Work out the finished part from the listing and answer in its coordinate system (mm). A direction names the side the tool comes from. Coordinates: 2 decimals unless noted, no trailing zeros. Order: outer loops, then holes, each group sorted by start corner. A loop starts at its lowest first (then second) coordinate and runs counter-clockwise, first axis right, second up. Notation, with made-up numbers: M -25,52.5 L -21,52.5 A7 ccw -21,59.5 Z; hole C 40.25,-34.75 d2. An arc over 180 degrees is marked long. Use a Markdown table: item, result.
from build123d import *

# Parameters (mm, degrees)
SKETCH1_R           = 2
BOSS_EXTRUDE1_DEPTH = 2
SKETCH2_W           = 54.569155846
SKETCH2_H           = 2
BOSS_EXTRUDE2_DEPTH = 10
SKETCH3_R           = 1.5
CUT_EXTRUDE1_DEPTH  = 73.112758927
SKETCH4_W           = 19.5
SKETCH4_H           = 5
SKETCH4_W_2         = 10
SKETCH4_H_2         = 4
CUT_EXTRUDE2_DEPTH  = 2.5
SKETCH5_W           = 19.5
SKETCH5_H           = 2
CUT_EXTRUDE3_DEPTH  = 4.5
FILLET1_R           = 1.5
FILLET2_R           = 0.5


with BuildPart() as part:
    # Sketch1 → Boss-Extrude1 (new body)
    with BuildSketch(Plane.XY):
        Polygon((0, 0), (21, -11), (27.728873239, -11), (34, -11), (34, -2), (40.5, 3), (63.5, 3), (63.5, 16), (61.378679656, 18.121320344), (61.378679656, 21), (6.80952381, 21), (0, 8), align=None)
        with Locations((26, -6.25)):
            Circle(SKETCH1_R, mode=Mode.SUBTRACT)
        with Locations((47, 6.5)):
            Circle(SKETCH1_R, mode=Mode.SUBTRACT)
        with Locations((60, 6.5)):
            Circle(SKETCH1_R, mode=Mode.SUBTRACT)
        with Locations((7.5, 16)):
            Circle(SKETCH1_R, mode=Mode.SUBTRACT)
    extrude(amount=BOSS_EXTRUDE1_DEPTH)

    # Sketch2 → Boss-Extrude2 (add)
    with BuildSketch(Plane.XY.offset(2)):
        with Locations((34.094101733, 20)):
            Rectangle(SKETCH2_W, SKETCH2_H)
    extrude(amount=BOSS_EXTRUDE2_DEPTH)

    # Sketch3 → Cut-Extrude1 (cut, through all)
    with BuildSketch(Plane(origin=(0, 21, 0), x_dir=(1, 0, 0), z_dir=(0, 1, 0))):
        with Locations(Location((52.878679656, -7.5, 0), (0, 0, 270))):
            Circle(SKETCH3_R)
        with Locations(Location((14.878679656, -7.5, 0), (0, 0, 270))):
            Circle(SKETCH3_R)
        Polygon((6.80952381, -2), (11.30952381, -12), (6.80952381, -12), align=None)
    extrude(amount=-CUT_EXTRUDE1_DEPTH, mode=Mode.SUBTRACT)

    # Sketch4 → Cut-Extrude2 (cut)
    with BuildSketch(Plane(origin=(0, 21, 0), x_dir=(1, 0, 0), z_dir=(0, 1, 0))):
        with Locations((27.628679656, -2.5)):
            Rectangle(SKETCH4_W, SKETCH4_H)
        with Locations((50.878679656, -2)):
            Rectangle(SKETCH4_W_2, SKETCH4_H_2)
    extrude(amount=-CUT_EXTRUDE2_DEPTH, mode=Mode.SUBTRACT)

    # Sketch5 → Cut-Extrude3 (cut)
    with BuildSketch(Plane(origin=(0, 18.5, 0), x_dir=(1, 0, 0), z_dir=(0, 1, 0))):
        with Locations((27.628679656, -1)):
            Rectangle(SKETCH5_W, SKETCH5_H)
    extrude(amount=-CUT_EXTRUDE3_DEPTH, mode=Mode.SUBTRACT)

    # Fillet1
    fillet1_edges = [part.edges().sort_by_distance(p)[0] for p in [
        (58.628679656, 21, 0),
        (0, 8, 1),
        (61.378679656, 18.121320344, 1),
        (63.5, 16, 1),
        (63.5, 3, 1),
        (40.5, 3, 1),
        (34, -2, 1),
        (34, -11, 1),
        (21, -11, 1),
        (0, 0, 1),
        (61.378679656, 20, 12),
        (11.30952381, 20, 12),
        (41.628679656, 21, 0),
        (12.344101733, 21, 0),
    ]]
    fillet(fillet1_edges, radius=FILLET1_R)

    # Fillet2
    fillet2_edges = [part.edges().sort_by_distance(p)[0] for p in [
        (37.378679656, 20, 5),
        (37.378679656, 14, 1),
        (55.878679656, 20, 4),
        (45.878679656, 20, 4),
        (45.878679656, 18.5, 1),
        (55.878679656, 18.5, 1),
        (17.878679656, 14, 1),
        (17.878679656, 20, 5),
    ]]
    fillet(fillet2_edges, radius=FILLET2_R)


solid = part.part
(1) A cutting plane is placed at A-A (x = 47). Determine the outline of the cut face in (y, z), then the cut area to 3 significant figures.
Conclusion:
| item | result |
|---|---|
| outline | M 3,0 L 4.5,0 L 4.5,2 L 3,2 Z; M 8.5,0 L 18.5,0 L 18.5,2 L 8.5,2 Z; M 19,4 L 21,4 L 21,12 L 19,12 Z |
| area | 39.0 mm2 |
(2) Determine the mould class of faces 1 (the flat face through (61.379, 20, 5)), 2 (the flat face through (37.379, 18.5, 1.8)), 3 (the flat face through (31, 5, 2)), 4 (the cylindrical face through (0.223, 0.121, 1.014)) for opening direction X: pulls with the +X half, pulls with the -X half, needs draft (parallel to the pull), parting line crosses it, or undercut.
Conclusion:
| item | result |
|---|---|
| face 1 | pulls with the +X half |
| face 2 | undercut |
| face 3 | needs draft |
| face 4 | pulls with the -X half |
(3) A cutting plane is placed at C-C (y = -5.5). Determine the outline of the cut face in (x, z), then the cut area to 3 significant figures.
Conclusion:
| item | result |
|---|---|
| outline | M 10.5,0 L 24.15,0 L 24.15,2 L 10.5,2 Z; M 27.85,0 L 34,0 L 34,2 L 27.85,2 Z |
| area | 39.6 mm2 |
(4) Straight lines are drawn through the part: L1, parallel to X at y = 5.5, z = 1; L2, parallel to Z at x = 39.5, y = 14; L3, parallel to Y at x = 16.5, z = 7.5. For each, find the intervals that lie inside material, in ascending order.
Conclusion:
| item | result |
|---|---|
| L1 | 0 to 45.27, 48.73 to 58.27, 61.73 to 63.5 |
| L2 | 0 to 2 |
| L3 | 19 to 21 |
(5) Which of the six approach directions +Z, -Z, +X, -X, +Y, -Y give full straight-line access (tool end or side, diameter ignored) to faces 5 (the flat face through (27, 14, 1)), 6 (the flat face through (45.879, 20, 2)), 7 (the flat face through (51, 3, 1))?
Conclusion:
| item | result |
|---|---|
| face 5 | +Z, -Z, +Y |
| face 6 | -Z, +Y |
| face 7 | +Z, -Z, +X, -Y |
(6) Given P1, Ø2, axis at y = -5.5, z = 1.5, coming from the +X side; P2, Ø2, axis at x = 24.5, z = 3.5, coming from the -Y side; P3, Ø1.6, axis at x = 51, y = 20, coming from the -Z side; P4, Ø4, axis at y = -4, z = 1.5, coming from the +X side, each flat-ended and moving along its own axis, determine where each tip first touches the part or whether it passes through.
Conclusion:
| item | result |
|---|---|
| P1 | x = 34 |
| P2 | through |
| P3 | z = 4 |
| P4 | x = 34.19 |
(7) A cutting plane is placed at B-B (y = 6.5). Determine the outline of the cut face in (x, z), then the cut area to 3 significant figures.
Conclusion:
| item | result |
|---|---|
| outline | M 0,0 L 45,0 L 45,2 L 0,2 Z; M 49,0 L 58,0 L 58,2 L 49,2 Z; M 62,0 L 63.5,0 L 63.5,2 L 62,2 Z |
| area | 111 mm2 |
(8) A cutting plane is placed at D-D (x = 7.5). Determine the outline of the cut face in (y, z), then the cut area to 3 significant figures.
Conclusion:
| item | result |
|---|---|
| outline | M -3.93,0 L 14,0 L 14,2 L -3.93,2 Z; M 18,0 L 19.5,0 A1.5 ccw 21,1.5 L 21,3.53 L 19,3.53 L 19,2 L 18,2 Z |
| area | 44.4 mm2 |
